Autodesk Inventor part; units mm, degrees
ref_plane "YZ Plane" through (0, 0, 0) normal (1, 0, 0) x (0, 1, 0)
ref_plane "XZ Plane" through (0, 0, 0) normal (0, 1, 0) x (-1, 0, 0)
ref_plane "XY Plane" through (0, 0, 0) normal (0, 0, 1) x (1, 0, 0)
sketch "Sketch1" plane through (0, 0, 0) normal (0, 0, 1) x (1, 0, 0)
  line L0 (3, 0) -> (40.64, 0)
  line L1 (37.65, 31.8) -> (0, 31.8)
  line L2 (0, 31.8) -> (0, 3)
  line L3 (37.65, 31.8) -> (40.65, 28.8)
  line L4 (3, 0) -> (0, 3)
  line L5 (40.65, 3) -> (37.65, 0)
  line L6 (40.65, 28.8) -> (40.65, 3)
  point P0 (0, 0)
  dimension "d4" = 3
  dimension "d5" = 45
  dimension "d6" = 45
  dimension "d7" = 3
  dimension "d8" = 31.8
  dimension "d9" = 40.65
  dimension "d10" = 3
extrude "Extrusion1" add sketch "Sketch1" along normal blind 1.651
sketch "Sketch2" plane through (0, 0, 1.651) normal (0, 0, 1) x (1, 0, 0)
  line L0 (2.418, 29.87) -> (38.232, 29.87)
  line L1 (38.232, 29.87) -> (38.232, 1.93)
  line L2 (38.232, 1.93) -> (2.418, 1.93)
  line L3 (2.418, 1.93) -> (2.418, 29.87)
  line L4 (0, 31.8) -> (0, 3)
  line L5 (3, 0) -> (37.65, 0)
  line L6 (40.65, 3) -> (40.65, 28.8)
  point P0 (0, 0)
  point P1 (0, 17.4)
  point P2 (20.325, 1.93)
  point P3 (20.325, 0)
  point P4 (38.232, 15.9)
  point P5 (40.65, 15.9)
  dimension "d13" = 27.94
  dimension "d14" = 35.814
extrude "Extrusion2" add sketch "Sketch2" along normal blind 1.65
sketch "Sketch3" plane through (0, 0, 3.301) normal (0, 0, 1) x (1, 0, 0)
  line L0 (4.925, 27.33) -> (35.725, 27.33)
  line L1 (35.725, 27.33) -> (35.725, 4.47)
  line L2 (35.725, 4.47) -> (4.925, 4.47)
  line L3 (4.925, 4.47) -> (4.925, 27.33)
  line L4 (2.418, 29.87) -> (2.418, 1.93)
  line L5 (3, 0) -> (37.65, 0)
  point P0 (0, 0)
  point P1 (4.925, 15.9)
  point P2 (2.418, 15.9)
  point P3 (20.325, 4.47)
  point P4 (20.325, 0)
  dimension "d17" = 22.86
  dimension "d18" = 30.8
extrude "Extrusion3" add sketch "Sketch3" along normal blind 2.83
sketch "Sketch4" plane through (0, 0, 6.131) normal (0, 0, 1) x (1, 0, 0)
  line L0 (11.825, 24.6) -> (28.825, 24.6)
  line L1 (33.025, 20.4) -> (33.025, 11.4)
  line L2 (28.825, 7.2) -> (11.825, 7.2)
  line L3 (7.625, 11.4) -> (7.625, 20.4)
  line L4 (4.925, 27.33) -> (4.925, 4.47)
  line L5 (2.418, 1.93) -> (38.232, 1.93)
  arc A0 (7.625, 11.4) -> (11.825, 7.2) centre (11.825, 11.4) ccw
  arc A1 (11.825, 24.6) -> (7.625, 20.4) centre (11.825, 20.4) ccw
  arc A2 (33.025, 20.4) -> (28.825, 24.6) centre (28.825, 20.4) ccw
  arc A3 (28.825, 7.2) -> (33.025, 11.4) centre (28.825, 11.4) ccw
  point P0 (0, 0)
  point P1 (7.625, 24.6)
  point P2 (33.025, 7.2)
  point P3 (7.625, 7.2)
  point P4 (7.625, 15.9)
  point P5 (4.925, 15.9)
  point P6 (20.325, 7.2)
  point P7 (20.325, 1.93)
  dimension "d21" = 17.4
  dimension "d22" = 25.4
  dimension "d23" = 4.2
extrude "Extrusion4" cut sketch "Sketch4" against normal blind 2.83
sketch "Sketch5" plane through (0, 0, 3.301) normal (0, 0, 1) x (1, 0, 0)
  line L0 (25.825, 11.775) -> (14.825, 11.775)
  line L1 (14.825, 11.775) -> (14.825, 20.025)
  line L2 (14.825, 20.025) -> (25.825, 20.025)
  line L3 (25.825, 20.025) -> (25.825, 11.775)
  line L4 (7.625, 11.4) -> (7.625, 20.4)
  line L5 (28.825, 7.2) -> (11.825, 7.2)
  point P0 (0, 0)
  point P1 (14.825, 15.9)
  point P2 (7.625, 15.9)
  point P3 (20.325, 11.775)
  point P4 (20.325, 7.2)
  dimension "d26" = 11
  dimension "d27" = 8.25
extrude "Extrusion5" add sketch "Sketch5" along normal blind 0.1
properties part number "DLP"
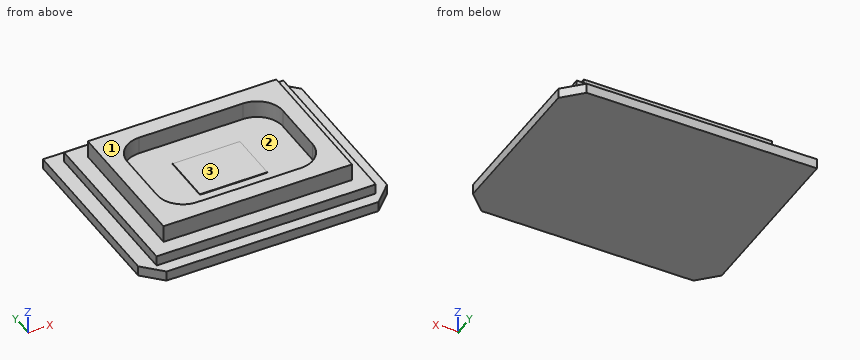
Input: part model. Units: mm. Frame: model coordinates. Face numbers are marked on the shaded views. Give positions to 0.01 mm unless a question says otherwise; leave off trailing zeros. Loops run counter-clockwise (first coordinate to the right, second up) from the corner with the lowest first, then second, coordinate; pieces in that order, holes last. Notation, with made-up numbers: M 45,-7.75 L 98,-7.75 A26 cw 98,13.25 Z; hole C 4.5,-21.5 d11. An arc over 180 degrees is marked long. Answer as CSV lines item,"result". Start each with the question number.
1. Pull-direction query (X, two-part tool) for the marked faces 1, 2 and 3; classes: released by +X, released by -X, zero draft, split by the parting line, or undercut.
2. Section B-B on x = 6. Return loops of the section in (y, z).
3. Section A-A on z = 5.5. Return loops of the section in (x, y) (3 decimals), plus the area to 3 significant figures.
4. Section D-D on y = 26.5. Return loops of the section in (x, z) (3 decimals).
5. Line query: L1, parallel to X at y = 18.5, z = 4.75 (3 decimals); L2, parallel to Y at x = 26, z = 3.5; L3, parallel to Z at x = 14, y = 16.5. Output: solid intervals per line, ascending.
6. Section C-C on y = 3.5. Return loops of the section in (x, z).
7. Pin query (flat end, axial travel): P1, Ø3, axis at x = 18.5, z = 4.5, coming from the -Y side; P2, Ø1.8, axis at y = 9, z = 3, coming from the -X side; P3, Ø2.5, axis at x = 17, z = 5.5, coming from the +Y side. Return the tip coordinate at first contact, or that it passes through.
Computed values:
1,face 1,"zero draft"
1,face 2,"undercut"
1,face 3,"undercut"
2,outline,"M 0,0 L 31.8,0 L 31.8,1.65 L 29.87,1.65 L 29.87,3.3 L 27.33,3.3 L 27.33,6.13 L 4.47,6.13 L 4.47,3.3 L 1.93,3.3 L 1.93,1.65 L 0,1.65 Z"
3,outline,"M 4.925,4.47 L 35.725,4.47 L 35.725,27.33 L 4.925,27.33 Z; hole M 7.625,11.4 A4.2 ccw 11.825,7.2 L 28.825,7.2 A4.2 ccw 33.025,11.4 L 33.025,20.4 A4.2 ccw 28.825,24.6 L 11.825,24.6 A4.2 ccw 7.625,20.4 Z"
3,area,"277 mm²"
4,outline,"M 0,0 L 40.65,0 L 40.65,1.651 L 38.232,1.651 L 38.232,3.301 L 35.725,3.301 L 35.725,6.131 L 4.925,6.131 L 4.925,3.301 L 2.418,3.301 L 2.418,1.651 L 0,1.651 Z"
5,L1,"x = 4.925 to 7.625, 33.025 to 35.725"
5,L2,"y = 4.47 to 7.2, 24.6 to 27.33"
5,L3,"z = 0 to 3.3"
6,outline,"M 0,0 L 40.65,0 L 40.65,1.65 L 38.23,1.65 L 38.23,3.3 L 2.42,3.3 L 2.42,1.65 L 0,1.65 Z"
7,P1,"stops at y = 1.93"
7,P2,"stops at x = 2.42"
7,P3,"stops at y = 27.33"
